Read the model definition and answer for the solid it produces. Units are mm, in the model's axes. A direction names the side the tool comes from. Coordinates: 2 decimals unless noted, no trailing zeros. Loops run counter-clockwise (first coordinate to the right, second up) from the corner with the lowest first, then second, coordinate; pieces in that order, holes last. Notation, with made-up numbers: (67.25, 49) -> (107.25, 49) arc R20 cw to (107.25, 58) -> close; hole circle Ø3 at (71.25, 20.25). An arc over 180 degrees is marked (long way). Answer in a Markdown table with one row per item.
```python
from build123d import *

# Parameters (mm, degrees)
SKETCH1_W               = 26
SKETCH1_H               = 37
BOSS_EXTRUDE1_DEPTH     = 5
SKETCH2_R               = 1.5
SKETCH2_R_2             = 5.5
CUT_EXTRUDE1_DEPTH      = 24.157072354
SKETCH3_W               = 26
SKETCH3_H               = 5
BOSS_EXTRUDE2_DEPTH     = 27
CUT_EXTRUDE2_DEPTH      = 36.217183306
CUT_EXTRUDE2_DEPTH_BACK = 36.217183306
SKETCH4_R               = 3.05
FILLET1_R               = 10
FILLET2_R               = 3
SKETCH5_W               = 2
SKETCH5_H               = 37
BOSS_EXTRUDE3_DEPTH     = 7
FILLET3_R               = 5


with BuildPart() as part:
    # Sketch1 → Boss-Extrude1 (new body)
    with BuildSketch(Plane(origin=(0, 0, 0), x_dir=(1, 0, 0), z_dir=(0, 1, 0))):
        Rectangle(SKETCH1_W, SKETCH1_H)
    extrude(amount=BOSS_EXTRUDE1_DEPTH)

    # Sketch2 → Cut-Extrude1 (cut, through all)
    with BuildSketch(Plane(origin=(0, 0, 0), x_dir=(1, 0, 0), z_dir=(0, 1, 0))):
        with Locations(Location((-5.75, 5.75, 0), (0, 0, 270))):
            Circle(SKETCH2_R)
        with Locations(Location((0, 0, 0), (0, 0, 270))):
            Circle(SKETCH2_R_2)
        with Locations(Location((5.75, 5.75, 0), (0, 0, 270))):
            Circle(SKETCH2_R)
        with Locations(Location((5.75, -5.75, 0), (0, 0, 270))):
            Circle(SKETCH2_R)
        with Locations(Location((-5.75, -5.75, 0), (0, 0, 270))):
            Circle(SKETCH2_R)
    extrude(amount=CUT_EXTRUDE1_DEPTH, mode=Mode.SUBTRACT)

    # Sketch3 → Boss-Extrude2 (add)
    with BuildSketch(Plane(origin=(0, 0, 0), x_dir=(1, 0, 0), z_dir=(0, 1, 0))):
        with Locations((0, 16)):
            Rectangle(SKETCH3_W, SKETCH3_H)
        with Locations((0, -16)):
            Rectangle(SKETCH3_W, SKETCH3_H)
    extrude(amount=BOSS_EXTRUDE2_DEPTH)

    # Sketch4 → Cut-Extrude2 (cut, two sides: drawn at the far end of the back side and taken through both)
    with BuildSketch(Plane.XY.offset(-CUT_EXTRUDE2_DEPTH_BACK)):
        with Locations((0, 17)):
            Circle(SKETCH4_R)
    extrude(amount=CUT_EXTRUDE2_DEPTH + CUT_EXTRUDE2_DEPTH_BACK, mode=Mode.SUBTRACT)

    # Fillet1
    fillet1_edges = [part.edges().sort_by_distance(p)[0] for p in [
        (-13, 27, -16),
        (13, 27, -16),
        (13, 27, 16),
        (-13, 27, 16),
    ]]
    fillet(fillet1_edges, radius=FILLET1_R)

    # Fillet2
    fillet2_edges = [part.edges().sort_by_distance(p)[0] for p in [
        (0, 5, -13.5),
        (0, 5, 13.5),
    ]]
    fillet(fillet2_edges, radius=FILLET2_R)

    # Sketch5 → Boss-Extrude3 (add)
    with BuildSketch(Plane(origin=(0, 0, 0), x_dir=(1, 0, 0), z_dir=(0, 1, 0))):
        with Locations((-12, 0)):
            Rectangle(SKETCH5_W, SKETCH5_H)
        with Locations((12, 0)):
            Rectangle(SKETCH5_W, SKETCH5_H)
    extrude(amount=BOSS_EXTRUDE3_DEPTH)

    # Fillet3
    # the kernel refuses this fillet: 5 mm, written as the material it adds along each edge
    with BuildSketch(Plane(origin=(13, 7, -13.328427125), x_dir=(0, 0, 1), z_dir=(-1, 0, 0))) as fillet3_piece_1:
        with BuildLine():
            CenterArc((4.828427125, 5), FILLET3_R, 180, 90)
            Line((-0.171572875, 5), (-0.671572875, 5))
            ThreePointArc((-0.671572875, 5), (-0.671572875, 1), (-0.471404521, -0.166666667))
            Line((-0.471404521, -0.166666667), (0, -0.5))
            Line((0, -0.5), (4.828427125, -0.5))
            Line((4.828427125, -0.5), (4.828427125, 0))
        make_face()
    extrude(amount=2)
    with BuildSketch(Plane(origin=(13, 7, 13.328427125), x_dir=(0, 0, -1), z_dir=(-1, 0, 0)), Plane(origin=(-11, 7, 13.328427125), x_dir=(0, 0, -1), z_dir=(-1, 0, 0))) as fillet3_piece_2:
        with BuildLine():
            CenterArc((4.828427125, -5), FILLET3_R, 90, 90)
            Line((-0.171572875, -5), (-0.671572875, -5))
            ThreePointArc((-0.671572875, -5), (-0.671572875, -1), (-0.471404521, 0.166666667))
            Line((-0.471404521, 0.166666667), (0, 0.5))
            Line((0, 0.5), (4.828427125, 0.5))
            Line((4.828427125, 0.5), (4.828427125, 0))
        make_face()
    extrude(amount=2)
    with BuildSketch(Plane(origin=(-11, 7, -13.328427125), x_dir=(0, 0.9994117743909562, -0.03429439033895371), z_dir=(-1, 0, 0))) as fillet3_piece_3:
        with BuildLine():
            CenterArc((4.831470907, -4.997058872), FILLET3_R, 88.034690809, 90)
            Line((-0.165587965, -4.82558692), (-0.665293852, -4.808439725))
            Line((-0.665293852, -4.808439725), (-0.499705887, 0.017147195))
            Line((-0.499705887, 0.017147195), (-0.150402098, 0.47684296))
            ThreePointArc((-0.150402098, 0.47684296), (1.022442957, 0.636883449), (5.020090054, 0.499705887))
            Line((5.020090054, 0.499705887), (5.002942859, 0))
        make_face()
    extrude(amount=2)


solid = part.part
```
1. A tool of negligible diameter and unlimited length cuts with its end or side. For faces 1 (the flat face through (12, 7, 0)), 2 (the cylindrical face through (-10.15, 23.99, 15.96)), from which of +Z, -Z, +X, -X, +Y, -Y can it reach the whole face along a straight path? Write none if from no direction.
A:
| item | result |
|---|---|
| face 1 | +X, -X, +Y |
| face 2 | +Z, -Z, -X, +Y |
2. A cutting plane is placed at A-A on z = 0. Give the vertices of the cut face in (x, y).
A:
| item | result |
|---|---|
| outline | (-13, 0) -> (-5.5, 0) -> (-5.5, 5) -> (-11, 5) -> (-11, 7) -> (-13, 7) -> close; (5.5, 0) -> (13, 0) -> (13, 7) -> (11, 7) -> (11, 5) -> (5.5, 5) -> close |
3. A cutting plane is placed at B-B on z = -14. Give the vertices of the cut face in (x, y), and give its area (3 significant figures).
A:
| item | result |
|---|---|
| outline | (-13, 0) -> (13, 0) -> (13, 17) arc R10 ccw to (3, 27) -> (-3, 27) arc R10 ccw to (-13, 17) -> close; hole circle Ø6.1 at (0, 17) |
| area | 630 mm2 |
4. A cutting plane is placed at D-D on y = 14.75. Give the vertices of the cut face in (x, z).
A:
| item | result |
|---|---|
| outline | (-13, -18.5) -> (-2.06, -18.5) -> (-2.06, -13.5) -> (-13, -13.5) -> close; (-13, 13.5) -> (-2.06, 13.5) -> (-2.06, 18.5) -> (-13, 18.5) -> close; (2.06, -18.5) -> (13, -18.5) -> (13, -13.5) -> (2.06, -13.5) -> close; (2.06, 13.5) -> (13, 13.5) -> (13, 18.5) -> (2.06, 18.5) -> close |
5. The mould has two halves that part along X. Classify faces 3 (the cylindrical face through (-5.37, 2.46, -1.19)), 4 (the flat face through (0, 27, 16)), 5 (the flat face through (0, 5, -7)), 6 (the flat face through (13, 6, 0)): pulls with the +X half, pulls with the -X half, needs draft (parallel to the pull), parting line crosses it, or undercut.
A:
| item | result |
|---|---|
| face 3 | undercut |
| face 4 | needs draft |
| face 5 | undercut |
| face 6 | pulls with the +X half |
6. Given pin 1 Ø3.5 at (x, z) = (-5.75, -5.75) entering from -Y; pin 2 Ø8 at (y, z) = (24, -14.5) entering from +X; pin 3 Ø2 at (x, z) = (-12, 3.5) entering from +Y; pin 4 Ø3.5 at (x, z) = (5.75, 5.75) entering from +Y, each flat-ended and moving along its own axis, determine where each tip first touches the part or whether it passes through.
A:
| item | result |
|---|---|
| pin 1 | stops at y = 0 |
| pin 2 | stops at x = 12.54 |
| pin 3 | stops at y = 7 |
| pin 4 | stops at y = 5 |
7. A cutting plane is placed at C-C on x = 0. Give the vertices of the cut face in (y, z).
A:
| item | result |
|---|---|
| outline | (0, -18.5) -> (13.95, -18.5) -> (13.95, -13.5) -> (8, -13.5) arc R3 cw to (5, -10.5) -> (5, -5.5) -> (0, -5.5) -> close; (0, 5.5) -> (5, 5.5) -> (5, 10.5) arc R3 cw to (8, 13.5) -> (13.95, 13.5) -> (13.95, 18.5) -> (0, 18.5) -> close; (20.05, -18.5) -> (27, -18.5) -> (27, -13.5) -> (20.05, -13.5) -> close; (20.05, 13.5) -> (27, 13.5) -> (27, 18.5) -> (20.05, 18.5) -> close |
8. Find the intervals of material crossed by probe 1 along Z at (x, y) = (-5.75, 2.75); probe 2 along X at (y, z) = (3, 5.75); probe 3 along Z at (x, y) = (10.5, 12), in increasing order.
A:
| item | result |
|---|---|
| probe 1 | z = -18.5 to -7.25, -4.25 to 4.25, 7.25 to 18.5 |
| probe 2 | x = -13 to -7.25, -4.25 to 4.25, 7.25 to 13 |
| probe 3 | z = -18.5 to -13.5, 13.5 to 18.5 |
